The model under review builds one solid part; all positions refer to its coordinate system, in mm. A direction names the side the tool comes from. Coordinates: 2 decimals unless noted, no trailing zeros. Write each loop counter-clockwise with the first axis right and the second up, starting at its lowest first coordinate (ties: lowest second). Pieces come first, ordered by that corner, then holes.
```python
from build123d import *

# Parameters (mm, degrees)
SKETCH1_W           = 67.8
SKETCH1_H           = 72.3
BOSS_EXTRUDE1_DEPTH = 1.6
SKETCH3_W           = 10
SKETCH3_H           = 56.699897886
BOSS_EXTRUDE2_DEPTH = 4
SKETCH4_W           = 8
SKETCH4_H           = 28.525313837
BOSS_EXTRUDE3_DEPTH = 10
SKETCH5_R           = 5
BOSS_EXTRUDE4_DEPTH = 17
SKETCH6_W           = 30
SKETCH6_H           = 59.3
BOSS_EXTRUDE5_DEPTH = 10


with BuildPart() as part:
    # Sketch1 → Boss-Extrude1 (new body)
    with BuildSketch(Plane.XY):
        with Locations((-4.278640777, 17.784757282)):
            Rectangle(SKETCH1_W, SKETCH1_H)
    extrude(amount=BOSS_EXTRUDE1_DEPTH)

    # Sketch3 → Boss-Extrude2 (add)
    with BuildSketch(Plane.XY.offset(1.6)):
        with Locations((-8.178640777, 18.484808339)):
            Rectangle(SKETCH3_W, SKETCH3_H)
    extrude(amount=BOSS_EXTRUDE2_DEPTH)

    # Sketch4 → Boss-Extrude3 (add)
    with BuildSketch(Plane.XY.offset(1.6)):
        with Locations((-27.178640777, 19.672100364)):
            Rectangle(SKETCH4_W, SKETCH4_H)
    extrude(amount=BOSS_EXTRUDE3_DEPTH)

    # Sketch5 → Boss-Extrude4 (add)
    with BuildSketch(Plane.XY.offset(1.6)):
        with Locations((-30.478640777, 39.934757282)):
            Circle(SKETCH5_R)
    extrude(amount=BOSS_EXTRUDE4_DEPTH)

    # Sketch6 → Boss-Extrude5 (add)
    with BuildSketch(Plane(origin=(0, 0, 0), x_dir=(-1, 0, 0), z_dir=(0, 0, -1))):
        with Locations((8.278640777, 16.984757282)):
            Rectangle(SKETCH6_W, SKETCH6_H)
    extrude(amount=BOSS_EXTRUDE5_DEPTH)


solid = part.part
```
Item 1: Mouldability with a two-part tool opening along X and no side actions: class faces 4 (the face through (-3.179, 18, 4)), 5 (the face through (-23.179, 19, 7)), 6 (the face through (-5, 53.935, 1)) as pulls with the +X half, pulls with the -X half, needs draft (parallel to the pull), parting line crosses it, or undercut.
Solved:
face 4: pulls with the +X half
face 5: undercut
face 6: needs draft
Item 2: Take a section at D-D, the plane z = -2.5. Write out the cut boundary in (x, y).
Solved:
outline: (-23.28, -12.67) - (6.72, -12.67) - (6.72, 46.63) - (-23.28, 46.63) - close
Item 3: To check wall thickness, follow line 1 along X through (y, z) = (43, -3.25); line 2 along Y through (x, z) = (-16.5, -4.75); line 3 along Z through (x, y) = (-6, 25). State the ranges of each line that lie inside material, in increasing order.
Solved:
line 1: x = -23.28 to 6.72
line 2: y = -12.67 to 46.63
line 3: z = -10 to 5.6
Item 4: Take a section at B-B, the plane y = 26.5. Write out the cut boundary in (x, z), plus the area to 3 significant figures.
Solved:
outline: (-38.18, 0) - (-23.28, 0) - (-23.28, -10) - (6.72, -10) - (6.72, 0) - (29.62, 0) - (29.62, 1.6) - (-3.18, 1.6) - (-3.18, 5.6) - (-13.18, 5.6) - (-13.18, 1.6) - (-23.18, 1.6) - (-23.18, 11.6) - (-31.18, 11.6) - (-31.18, 1.6) - (-38.18, 1.6) - close
area: 528 mm2
Item 5: For pin 1 (8 mm diameter, centred on x = -8, y = 29.5, fed in from +Z); pin 2 (5 mm diameter, centred on x = 15.5, y = 25, fed in from +Z); pin 3 (4.5 mm diameter, centred on y = 22.5, z = 4, fed in from -X), all flat-tipped, find the tip position at first contact; note any pin that passes through.
Solved:
pin 1: stops at z = 5.6
pin 2: stops at z = 1.6
pin 3: stops at x = -31.18
Item 6: Take a section at A-A, the plane x = -17.5. Write out the cut boundary in (y, z), plus the area to 3 significant figures.
Solved:
outline: (-18.37, 0) - (-12.67, 0) - (-12.67, -10) - (46.63, -10) - (46.63, 0) - (53.93, 0) - (53.93, 1.6) - (-18.37, 1.6) - close
area: 709 mm2
Item 7: Take a section at C-C, the plane z = 9. Write out the cut boundary in (x, y), plus the area to 3 significant figures.
Solved:
outline: circle Ø10 at (-30.48, 39.93); (-31.18, 5.41) - (-23.18, 5.41) - (-23.18, 33.93) - (-31.18, 33.93) - close
area: 307 mm2
Item 8: Machinability: for faces 1 (the face through (6.721, 17, -5)), 2 (the face through (-27, 20, 11.6)), 3 (the face through (-31.13, 44.892, 9.981)), which of the approach directions +Z, -Z, +X, -X, +Y, -Y give a long, thin tool a straight path to every point of the face, cutting with its end or side? Answer none if there is none.
Solved:
face 1: -Z, +X, +Y, -Y
face 2: +Z, +X, -X, -Y
face 3: +Z
